For this review, take the finished solid that the model builds, in its own axes (mm). Give positions to 0.01 mm unless a question says otherwise; leave off trailing zeros. Loops run counter-clockwise (first coordinate to the right, second up) from the corner with the lowest first, then second, coordinate; pieces in that order, holes last. Notation, with made-up numbers: (64, 66) - (71, 66) arc R5 cw to (71, 75) - close; hole circle Ø4 at (15, 22.5). An arc over 180 degrees is marked (long way). Put each result on its own line as item: value.
Autodesk Inventor part; units mm, degrees
ref_plane "Plano inicial" through (0, 0, 0) normal (0, 0, 1) x (1, 0, 0)
ref_plane "Plano final" through (0, 0, 700) normal (0, 0, 1) x (1, 0, 0)
ref_plane "YZ Plane" through (0, 0, 0) normal (1, 0, 0) x (0, 1, 0)
ref_plane "Plano inicial" through (0, 0, 0) normal (0, 0, 1) x (1, 0, 0)
ref_plane "Plano final" through (0, 0, 700) normal (0, 0, 1) x (1, 0, 0)
sketch "Rascunho" plane through (0, 0, 0) normal (0, 0, 1) x (1, 0, 0)
  line L0 (30, 0) -> (0, 0)
  line L1 (0, 0) -> (0, 30)
  line L2 (0, 30) -> (2, 30)
  line L3 (5, 27) -> (5, 10)
  line L4 (10, 5) -> (27, 5)
  line L5 (30, 2) -> (30, 0)
  line L6 (0, -11.0414) -> (0, 31.5385) construction
  line L7 (-11.0414, 0) -> (31.5385, 0) construction
  arc A0 (5, 10) -> (10, 5) centre (10, 10) ccw
  arc A1 (5, 27) -> (2, 30) centre (2, 27) ccw
  arc A2 (30, 2) -> (27, 5) centre (27, 2) ccw
  line L8 (0, 62.9539) -> (0, -23.374) construction
  line L9 (-23.374, 0) -> (62.9539, 0) construction
  point P0 (5, 30)
  point P1 (5, 5)
  point P2 (30, 5)
  dimension "d0" = 30
  dimension "d1" = 30
  dimension "d2" = 5
  dimension "d3" = 5
  dimension "d8" = 5
  dimension "d9" = 3
  dimension "d10" = 0
  dimension "d11" = 0
extrude "Corpo" add sketch "Rascunho" along normal up to surface (700 mm away) from surface at 0
sketch "Sketch3" plane through (0, 0, 0) normal (0, 0, 1) x (1, 0, 0)
  line L0 (0, 0) -> (10, 0)
ref_plane "Work Plane3" through (0, 0, 0) normal (0, -1, 0) x (1, 0, 0)
sketch "Sketch4" plane through (0, 0, 0) normal (0, -1, 0) x (1, 0, 0)
  line L0 (-2, 0) -> (12, 0)
  line L1 (-2, 700) -> (12, 700)
  dimension "d15" = 700
equation "\"d0\" = G_H"
equation "\"d1\" = G_H"
equation "\"d2\" = G_T"
equation "\"d3\" = G_T"
equation "\"d8\" = G_IR"
equation "\"d9\" = G_ER"
equation "\"d4\" = G_L"
equation "\"G_H\" = 30"
equation "\"G_T\" = 5"
equation "\"G_ER\" = 3"
equation "\"G_IR\" = 5"
equation "\"G_L\" = d15"
equation "\"ex\" = 0"
equation "\"G_OFFSET_START\" = 0"
equation "\"G_OFFSET_END\" = 0"
properties part number "IS 808 - ISA 3030 - 700" material "Aço, suave"
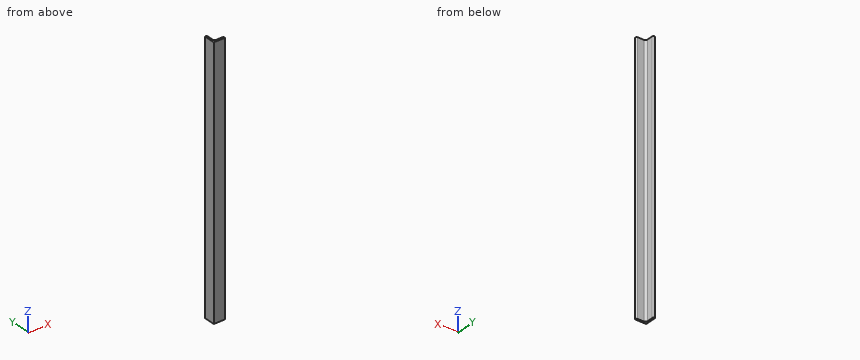
1) Take a section at B-B on x = 16. State the section outline as (y, z) points.
Geometry check:
outline: (0, 0) - (5, 0) - (5, 700) - (0, 700) - close
2) Take a section at A-A on z = 645.5. State the section outline as (x, y) points.
Geometry check:
outline: (0, 0) - (30, 0) - (30, 2) arc R3 ccw to (27, 5) - (10, 5) arc R5 cw to (5, 10) - (5, 27) arc R3 ccw to (2, 30) - (0, 30) - close
3) Insertion check: pin 1 Ø5 at (x, y) = (5.5, 9.5) entering from +Z; pin 2 Ø12 at (x, y) = (22.5, 16.5) entering from -Z; pin 3 Ø4 at (x, z) = (5, 142.5) entering from +Y; pin 4 Ø2 at (x, z) = (10, 441.5) entering from +Y. Each pin has a flat end and moves straight along its axis. Give the tip position at first contact, or say it passes through.
Geometry check:
pin 1: stops at z = 700
pin 2: passes through
pin 3: stops at y = 29.83
pin 4: stops at y = 5.1
4) Wall thickness on line 1 (X direction, y = 26, z = 236.5); line 2 (Y direction, x = 2.75, z = 512): over which ranges is each line inside the solid? List them lowest first.
Geometry check:
line 1: x = 0 to 5
line 2: y = 0 to 29.9
